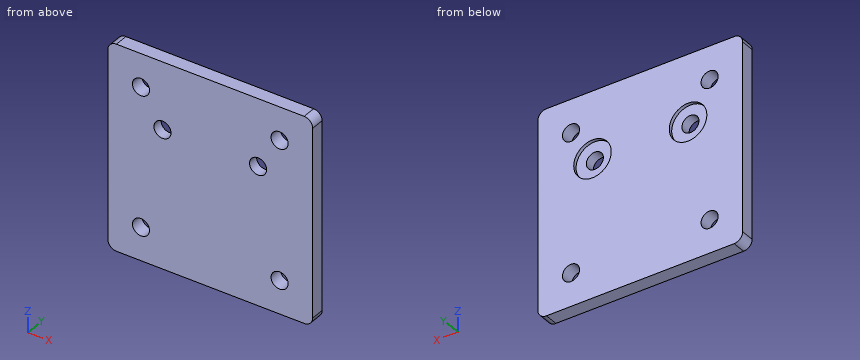
from build123d import *

# Parameters (mm, degrees)
F0_W     = 60
F0_H     = 60
F1_DEPTH = 4
F2_D     = 5
F4_D     = 5
F5_R     = 5.5
F6_DEPTH = 1
F7_R     = 2.5


with BuildPart() as f1:
    # F0 (on Front) → F1 (new body)
    with BuildSketch(Plane.XZ):
        Rectangle(F0_W, F0_H)
    extrude(amount=F1_DEPTH)

    # F2 (through all)
    with Locations(Plane(origin=(0, 0, 0), x_dir=(1, 0, 0), z_dir=(0, 1, 0))):
        with Locations((-20.3, -20.3), (20.3, -20.3), (20.3, 20.3), (-20.3, 20.3)):
            Hole(F2_D / 2)

    # F4 (through all)
    with Locations(Plane.XZ.offset(4)):
        with Locations((-14, 10.35), (14, 10.35)):
            Hole(F4_D / 2)

    # F5 (on face) → F6 (cut)
    with BuildSketch(Plane.XZ):
        with Locations((14, 10.35)):
            Circle(F5_R)
        with Locations((-14, 10.35)):
            Circle(F5_R)
    extrude(amount=F6_DEPTH, mode=Mode.SUBTRACT)

    # F7
    f7_edges = [f1.edges().sort_by_distance(p)[0] for p in [
        (30, -2, 30),
        (30, -2, -30),
        (-30, -2, -30),
        (-30, -2, 30),
    ]]
    fillet(f7_edges, radius=F7_R)


solid = f1.part
Input: part model. Units: mm. Frame: model coordinates. Give positions to 0.01 mm unless a question says otherwise; leave off trailing zeros. Order: outer loops, then holes, each group sorted by start corner. A loop starts at its lowest first (then second) coordinate and runs counter-clockwise, first axis right, second up. Notation, with made-up numbers: (34.5, 69.5) -> (89.5, 69.5) arc R18 ccw to (89.5, 84.5) -> close; hole circle Ø7 at (-3, -24). An arc over 180 degrees is marked (long way). Use one line per item in the form item = value.
1) Section D-D, the plane x = -20.3. Return loops of the section in (y, z), and give its area (3 significant figures).
Response values:
outline = (-4, -30) -> (0, -30) -> (0, -22.8) -> (-4, -22.8) -> close; (-4, -17.8) -> (0, -17.8) -> (0, 17.8) -> (-4, 17.8) -> close; (-4, 22.8) -> (0, 22.8) -> (0, 30) -> (-4, 30) -> close
area = 200 mm^2
2) Section C-C, the plane y = -2.65. Return loops of the section in (x, z).
Response values:
outline = (-30, -27.5) arc R2.5 ccw to (-27.5, -30) -> (27.5, -30) arc R2.5 ccw to (30, -27.5) -> (30, 27.5) arc R2.5 ccw to (27.5, 30) -> (-27.5, 30) arc R2.5 ccw to (-30, 27.5) -> close; hole circle Ø5 at (-20.3, -20.3); hole circle Ø5 at (-20.3, 20.3); hole circle Ø5 at (-14, 10.35); hole circle Ø5 at (14, 10.35); hole circle Ø5 at (20.3, -20.3); hole circle Ø5 at (20.3, 20.3)
3) First-contact query: pin 1 Ø6 at (x, z) = (-20.3, 20.3) entering from +Y. Flat tip, straight axial feed; report the tip coordinate or a pass-through.
Response values:
pin_1 = 0
4) Section A-A, the plane z = 10.35. Return loops of the section in (x, y).
Response values:
outline = (-30, -4) -> (-16.5, -4) -> (-16.5, -1) -> (-19.5, -1) -> (-19.5, 0) -> (-30, 0) -> close; (-11.5, -4) -> (11.5, -4) -> (11.5, -1) -> (8.5, -1) -> (8.5, 0) -> (-8.5, 0) -> (-8.5, -1) -> (-11.5, -1) -> close; (16.5, -4) -> (30, -4) -> (30, 0) -> (19.5, 0) -> (19.5, -1) -> (16.5, -1) -> close
5) Section B-B, the plane x = -14. Return loops of the section in (y, z), and give its area (3 significant figures).
Response values:
outline = (-4, -30) -> (0, -30) -> (0, 4.85) -> (-1, 4.85) -> (-1, 7.85) -> (-4, 7.85) -> close; (-4, 12.85) -> (-1, 12.85) -> (-1, 15.85) -> (0, 15.85) -> (0, 30) -> (-4, 30) -> close
area = 214 mm^2
6) Line query: probe 1 along Z at (x, y) = (-20.3, -2.05); probe 2 along Z at (x, y) = (-14, -3.1). Output: solid intervals per line, ascending.
Response values:
probe_1 = -30 to -22.8, -17.8 to 17.8, 22.8 to 30
probe_2 = -30 to 7.85, 12.85 to 30
